Could you check a few things on this model? Use its own coordinates, in mm. A direction names the side the tool comes from. Round coordinates to 2 decimals unless told otherwise and drop trailing zeros. Loops run counter-clockwise (first coordinate to the right, second up) from the corner with the lowest first, then second, coordinate; pieces in that order, holes last. Notation, with made-up numbers: M 80,78.5 L 135,78.5 A15 ccw 135,83.5 Z; hole C 5.25,68.25 d11. An arc over 180 degrees is marked long. Answer in a Markdown table with one row per item.
Autodesk Fusion 360 part; units mm, degrees
sketch "Esquisse1" plane through (0, 0, 0) normal (0, 0, 1) x (1, 0, 0)
  circle A0 centre (0, 0) radius 6.5
  circle A1 centre (0, 64) radius 6.5
  line L0 (0, 64) -> (0, 0)
  line L1 (0, 64) -> (6.5, 64)
  line L2 (0, 64) -> (-6.5, 64)
  line L3 (0, 0) -> (6.5, 0)
  line L4 (0, 0) -> (-6.5, 0)
  line L5 (6.5, 64) -> (6.5, 0)
  line L6 (-6.5, 64) -> (-6.5, 0)
  circle A2 centre (0, 64) radius 1.5
  circle A3 centre (0, 0) radius 1.5
  dimension "d1" = 13
  dimension "d2" = 13
  dimension "d3" = 64
  dimension "d4" = 3
  dimension "d5" = 3
extrude "Extrusion1" add sketch "Esquisse1" along normal blind 5 contours A0 L3 L4 A3 | A0 A1 L0 L6 | A0 L0 L4 A3 | A0 L0 L3 A3 | A0 A1 L0 L5 | A1 L0 L2 A2 | A1 L1 L2 A2 | A1 L0 L1 A2
sketch "Esquisse2" plane through (0, 0, 5) normal (0, 0, 1) x (-1, 0, 0)
  circle A0 centre (0, 0) radius 1.5
  circle A1 centre (0, -64) radius 1.5
  arc A2 (-6.5, -64) -> (6.5, -64) centre (0, -64) ccw
  line L0 (6.5, -64) -> (6.5, 0)
  arc A3 (6.5, 0) -> (-6.5, 0) centre (0, 0) ccw
  line L1 (-6.5, 0) -> (-6.5, -64)
  circle A4 centre (0, -64) radius 3.5
  circle A5 centre (0, -64) radius 1.5
  circle A6 centre (0, 0) radius 1.5
  circle A7 centre (0, 0) radius 3.5
  dimension "d8" = 3
  dimension "d9" = 7
  dimension "d10" = 3
  dimension "d11" = 7
extrude "Extrusion2" add sketch "Esquisse2" along normal blind 2 contours A4 | A7
1) I want a section at C-C, the plane y = 30.5. Please give me the cut outline in (x, z).
Computed:
| item | result |
|---|---|
| outline | M -6.5,0 L 6.5,0 L 6.5,5 L -6.5,5 Z |
2) Which directions (+Z, -Z, +X, -X, +Y, -Y) give clear straight access to the entire face, cutting with the end or side of a thin tool? Please do faces 1 (the face through (-1.88, 66.95, 5.99)), 2 (the face through (6.5, 32, 2)).
Computed:
| item | result |
|---|---|
| face 1 | +Z |
| face 2 | +Z, -Z, +X, +Y, -Y |
3) I need wall thicknesses on line 1 (Y direction, x = 0, z = 3.5); line 2 (X direction, y = 0, z = 2); line 3 (X direction, y = 0, z = 5.25). Which ranges of each line are inside material? Lowest first, please.
Computed:
| item | result |
|---|---|
| line 1 | y = -6.5 to -1.5, 1.5 to 62.5, 65.5 to 70.5 |
| line 2 | x = -6.5 to -1.5, 1.5 to 6.5 |
| line 3 | x = -3.5 to -1.5, 1.5 to 3.5 |
4) Will these pins go through, and if not, where does the flat tip stop? P1, Ø2.5, axis at x = 0, y = 0, coming from the -Z side; P2, Ø6.5, axis at x = -1.5, y = 33, coming from the +Z side.
Computed:
| item | result |
|---|---|
| P1 | passes through |
| P2 | stops at z = 5 |
5) I want a section at A-A, the plane z = 2.5. Please give me the cut outline in (x, y).
Computed:
| item | result |
|---|---|
| outline | M -6.5,0 A6.5 ccw 6.5,0 L 6.5,64 A6.5 ccw -6.5,64 Z; hole C 0,0 d3; hole C 0,64 d3 |
6) I want a section at D-D, the plane x = 5.75. Please give me the cut outline in (y, z), plus the area to 3 significant figures.
Computed:
| item | result |
|---|---|
| outline | M -3.03,0 L 67.03,0 L 67.03,5 L -3.03,5 Z |
| area | 350 mm² |
